from build123d import *

# Parameters (mm, degrees)
SKETCH1_W               = 100
SKETCH1_H               = 32
BOSS_EXTRUDE1_DEPTH     = 2
SKETCH2_W               = 100
SKETCH2_H               = 2
BOSS_EXTRUDE2_DEPTH     = 46
SKETCH3_W               = 100
SKETCH3_H               = 2
BOSS_EXTRUDE3_DEPTH     = 32
CUT_EXTRUDE1_DEPTH      = 117.292734081
CUT_EXTRUDE1_DEPTH_BACK = 117.292734081
SKETCH4_R               = 2.25
CUT_EXTRUDE2_DEPTH      = 117.292734081
CUT_EXTRUDE2_DEPTH_BACK = 117.292734081
SKETCH5_W               = 36
SKETCH5_H               = 32
SKETCH6_W               = 25
SKETCH6_H               = 20
CUT_EXTRUDE3_DEPTH      = 2
FILLET1_R               = 1


with BuildPart() as part:
    # Sketch1 → Boss-Extrude1 (new body)
    with BuildSketch(Plane(origin=(0, 0, 0), x_dir=(1, 0, 0), z_dir=(0, 1, 0))):
        with Locations((50, 16)):
            Rectangle(SKETCH1_W, SKETCH1_H)
    extrude(amount=BOSS_EXTRUDE1_DEPTH)

    # Sketch2 → Boss-Extrude2 (add)
    with BuildSketch(Plane.XZ):
        with Locations((50, -1)):
            Rectangle(SKETCH2_W, SKETCH2_H)
    extrude(amount=BOSS_EXTRUDE2_DEPTH)

    # Sketch3 → Boss-Extrude3 (add)
    with BuildSketch(Plane.XY):
        with Locations((50, -47)):
            Rectangle(SKETCH3_W, SKETCH3_H)
    extrude(amount=-BOSS_EXTRUDE3_DEPTH)

    # Sketch4 → Cut-Extrude1 (cut, two sides: drawn at the far end of the back side and taken through both)
    with BuildSketch(Plane(origin=(0, 2, 0), x_dir=(1, 0, 0), z_dir=(0, 1, 0)).offset(-CUT_EXTRUDE1_DEPTH_BACK)):
        with Locations(Location((7.6, 22.75, 0), (0, 0, 270))):
            Circle(SKETCH4_R)
        with Locations(Location((56.4, 22.75, 0), (0, 0, 270))):
            Circle(SKETCH4_R)
        with Locations(Location((56.4, 12.75, 0), (0, 0, 270))):
            Circle(SKETCH4_R)
        Polygon((52.2, 17.25), (59, 17.25), (59, 18.25), (52.2, 18.25), (52.2, 27.75), (11.8, 27.75), (11.8, 18.25), (5, 18.25), (5, 17.25), (11.8, 17.25), (11.8, 7.75), (52.2, 7.75), align=None)
        with Locations(Location((7.6, 12.75, 0), (0, 0, 270))):
            Circle(SKETCH4_R)
    extrude(amount=CUT_EXTRUDE1_DEPTH + CUT_EXTRUDE1_DEPTH_BACK, mode=Mode.SUBTRACT)

    # Sketch5 → Cut-Extrude2 (cut, two sides: drawn at the far end of the back side and taken through both)
    with BuildSketch(Plane.XZ.offset(48).offset(-CUT_EXTRUDE2_DEPTH_BACK)):
        with Locations((82, -16)):
            Rectangle(SKETCH5_W, SKETCH5_H)
    extrude(amount=CUT_EXTRUDE2_DEPTH + CUT_EXTRUDE2_DEPTH_BACK, mode=Mode.SUBTRACT)

    # Sketch6 → Cut-Extrude3 (cut)
    with BuildSketch(Plane(origin=(0, 0, -2), x_dir=(-1, 0, 0), z_dir=(0, 0, -1))):
        with Locations((-51.5, -36)):
            Rectangle(SKETCH6_W, SKETCH6_H)
    extrude(amount=-CUT_EXTRUDE3_DEPTH, mode=Mode.SUBTRACT)

    # Fillet1
    fillet1_edges = [part.edges().sort_by_distance(p)[0] for p in [
        (0, 1, -32),
        (0, -47, -32),
        (64, -47, -32),
        (64, 1, -32),
        (32, 0, -2),
        (19.5, -46, -2),
        (64, -47, 0),
        (64, -26, -1),
    ]]
    fillet(fillet1_edges, radius=FILLET1_R)


solid = part.part
Build history of the part. All positions in model axes, mm. A direction names the side the tool comes from. Coordinates: 2 decimals unless noted, no trailing zeros. Write each loop counter-clockwise with the first axis right and the second up, starting at its lowest first coordinate (ties: lowest second). Pieces come first, ordered by that corner, then holes.
(1) Cut at D-D on x = 20. List the corners of the cut face in (y, z), and give its area (3 significant figures).
(2) Mould opens along Y. For faces 1 (the flat face through (32, -48, -5)), 2 (the flat face through (24, -23, -2)), 3 (the flat face through (11.8, -47, -13)), 4 (the flat face through (32, 0, -31)) say: pulls with the +Y half, pulls with the -Y half, needs draft (parallel to the pull), parting line crosses it, or undercut.
(3) 3-axis set-ups, long thin cutter, end or side, ignore diameter. For faces 5 (the flat face through (32, 2, -6)), 6 (the flat face through (56, 1, -18.25)), 7 (the flat face through (51, -26, -1)): which of +Z, -Z, +X, -X, +Y, -Y reach the whole face in a straight line?
(4) Drill centre lines: line 1 (Z direction, x = 56.4, y = 1.65); line 2 (X direction, y = -47.45, z = -12.75); line 3 (Y direction, x = 5.5, z = -11). Where is each one in solid material? Low to high.
(5) Cut at A-A on x = 7.6. State how many separate pieces and enclosed holes the cut face has, and give its area (3 significant figures).
(6) Pin check, flat tip, straight feed: pin 1 Ø5 at (x, z) = (25, -25) entering from -Y. Stop position of the tip, or through.
(7) Cut at B-B on x = 53. List the corners of the cut face in (y, z).
Working result:
1. outline: (-48, -32) - (-46, -32) - (-46, -27.75) - (-48, -27.75) - close; (-48, -7.75) - (-46, -7.75) - (-46, -3) arc R1 cw to (-45, -2) - (-1, -2) arc R1 cw to (0, -3) - (0, -7.75) - (2, -7.75) - (2, 0) - (-48, 0) - close; (0, -32) - (2, -32) - (2, -27.75) - (0, -27.75) - close
1. area: 140 mm2
2. face 1: pulls with the -Y half
2. face 2: undercut
2. face 3: needs draft
2. face 4: undercut
3. face 5: +Z, -Z, +X, -X, +Y
3. face 6: +Y, -Y
3. face 7: +Z, -Z, +X
4. line 1: z = -32 to -25, -20.5 to -18.25, -17.25 to -15, -10.5 to 0
4. line 2: x = 0 to 5.35, 9.85 to 11.8, 52.2 to 54.15, 58.65 to 64
4. line 3: y = -48 to -46, 0 to 2
5. separate pieces: 7
5. enclosed holes: 0
5. area: 180 mm2
6. pin 1: passes through
7. outline: (-48, -32) - (-46, -32) - (-46, -18.25) - (-48, -18.25) - close; (-48, -17.25) - (-46, -17.25) - (-46, 0) - (-48, 0) - close; (-26, -2) - (-1, -2) arc R1 cw to (0, -3) - (0, -17.25) - (2, -17.25) - (2, 0) - (-26, 0) - close; (0, -32) - (2, -32) - (2, -18.25) - (0, -18.25) - close
